from build123d import *

# Parameters (mm, degrees)
SKETCH_1_R               = 5
EXTRUDE_1_DEPTH          = 15
SKETCH_2_R               = 3.55
CUT_EXTRUDE_1_DEPTH      = 3
SKETCH_3_R               = 3
CUT_EXTRUDE_2_DEPTH      = 10
CUT_EXTRUDE_3_DEPTH      = 5
CUT_EXTRUDE_3_DEPTH_BACK = 5
SKETCH_4_R               = 1


with BuildPart() as part:
    # Sketch 1 → Extrude 1 (new body)
    with BuildSketch(Plane(origin=(0, 0, 0), x_dir=(0, 0, -1), z_dir=(1, 0, 0))):
        Circle(SKETCH_1_R)
    extrude(amount=EXTRUDE_1_DEPTH)

    # Sketch 2 → Cut-Extrude 1 (cut)
    with BuildSketch(Plane(origin=(15, 0, 0), x_dir=(0, 0, -1), z_dir=(1, 0, 0))):
        Circle(SKETCH_2_R)
    extrude(amount=-CUT_EXTRUDE_1_DEPTH, mode=Mode.SUBTRACT)

    # Sketch 3 → Cut-Extrude 2 (cut)
    with BuildSketch(Plane.ZY):
        Circle(SKETCH_3_R)
    extrude(amount=-CUT_EXTRUDE_2_DEPTH, mode=Mode.SUBTRACT)

    # Sketch 4 → Cut-Extrude 3 (cut, two sides: drawn at the far end of the back side and taken through both)
    with BuildSketch(Plane.XY.offset(-CUT_EXTRUDE_3_DEPTH_BACK)):
        with Locations(Location((5, 0, 0), (0, 0, 180))):
            Circle(SKETCH_4_R)
    extrude(amount=CUT_EXTRUDE_3_DEPTH + CUT_EXTRUDE_3_DEPTH_BACK, mode=Mode.SUBTRACT)


solid = part.part
Design review of the part built by this model. Coordinates are the model's own, in mm. A direction names the side the tool comes from. Give positions to 0.01 mm unless a question says otherwise; leave off trailing zeros. Order: outer loops, then holes, each group sorted by start corner. A loop starts at its lowest first (then second) coordinate and runs counter-clockwise, first axis right, second up.
1. Add section B-B, the plane z = 4. State the section outline as (x, y) points, then the cut area to 3 significant figures.
Solution:
outline: (0, -3) - (15, -3) - (15, 3) - (0, 3) - close; hole circle Ø2 at (5, 0)
area: 86.9 mm2
2. Add section C-C, the plane z = 0. State the section outline as (x, y) points.
Solution:
outline: (0, -5) - (15, -5) - (15, -3.55) - (12, -3.55) - (12, 3.55) - (15, 3.55) - (15, 5) - (0, 5) - (0, 3) - (10, 3) - (10, -3) - (0, -3) - close
3. Mouldability with a two-part tool opening along Y and no side actions: class faces 4 (the flat face through (0, -3.3, 0.1)), 5 (the cylindrical face through (7.4, 1.5, -4.77)), 6 (the cylindrical face through (5, -1, 4)) as +Y half, -Y half, draft (parallel to the pull), parting line (faces both ways), or undercut.
Solution:
face 4: draft
face 5: parting line
face 6: undercut
4. For pin 1 Ø4 at (x, z) = (10.5, -2.5) entering from +Y; pin 2 Ø1.6 at (x, y) = (5, 0) entering from +Z; pin 3 Ø1 at (x, y) = (4, -2.5) entering from +Z; pin 4 Ø1.5 at (y, z) = (0.5, 1.5) entering from -X, all flat-tipped, find the tip position at first contact; note any pin that passes through.
Solution:
pin 1: stops at y = 4.97
pin 2: passes through
pin 3: stops at z = 4.58
pin 4: stops at x = 10
5. To check wall thickness, follow L1, parallel to Y at x = 6, z = 0; L2, parallel to Y at x = 13.2, z = 0; L3, parallel to X at y = -1.5, z = 0. State the ranges of each line that lie inside material, in increasing order.
Solution:
L1: y = -5 to -3, 3 to 5
L2: y = -5 to -3.55, 3.55 to 5
L3: x = 10 to 12
6. Add section D-D, the plane x = 12.25. State the section outline as (y, z) points, then the cut area to 3 significant figures.
Solution:
outline: circle Ø10 at (0, 0); hole circle Ø7.1 at (0, 0)
area: 38.9 mm2
7. Add section A-A, the plane x = 5. State the section outline as (y, z) points.
Solution:
outline: (-1, -4.9) - (-1, -2.83) arc R3 cw to (-1, 2.83) - (-1, 4.9) arc R5 ccw to start; (1, -4.9) arc R5 ccw to (1, 4.9) - (1, 2.83) arc R3 cw to (1, -2.83) - close
8. Tool access review of faces 1 (the flat face through (12, 0, 0)), 2 (the flat face through (10, 0, 0)), 3 (the cylindrical face through (6, 0, -4)): name each direction out of +Z, -Z, +X, -X, +Y, -Y from which nothing blocks a thin tool from reaching the whole face with its end or side.
Solution:
face 1: +X
face 2: -X
face 3: +Z, -Z
